Read the model definition and answer for the solid it produces. Units are mm, in the model's axes. A direction names the side the tool comes from. Give positions to 0.01 mm unless a question says otherwise; leave off trailing zeros. Order: outer loops, then holes, each group sorted by start corner. A loop starts at its lowest first (then second) coordinate and runs counter-clockwise, first axis right, second up. Notation, with made-up numbers: (-0.5, -22.75) - (15.5, -22.75) arc R16 cw to (15.5, -12.75) - close; hole circle Ø7 at (52, 12). An arc over 180 degrees is marked (long way). Use a Markdown table: item, result. Add a question column.
1. A cutting plane is placed at A-A on x = 0. Determine the outline of the cut face in (y, z) (1 decimal), and give its area (3 significant figures).
2. A cutting plane is placed at D-D on z = 0.75. Determine the outline of the cut face in (x, y) (3 decimals), and give its area (3 significant figures).
3. Which of the six approach directions +Z, -Z, +X, -X, +Y, -Y give full straight-line access (tool end or side, diameter ignored) to faces 4 (the cylindrical face through (-2.94, 0.13, -8.49)), 5 (the flat face through (-3.175, 0, -2)), 6 (the flat face through (0, 7, -3.048)), 7 (the flat face through (5, 0, 0))?
4. Consider L1, parallel to Y at x = 0, z = -1.95 (3 decimals); L2, parallel to X at y = 2, z = -2.75 (3 decimals); L3, parallel to Z at x = -3.75, y = 8.25. Determine where each line is inside the solid, lowest interval first.
5. Flat-ended cylindrical pins translate along their axes: P1, Ø3, axis at y = -1.5, z = -7.5, coming from the +X side; P2, Ø3.5, axis at x = 0, y = 6.477, coming from the +Z side; P3, Ø1, axis at x = 4.5, y = 5, coming from the -Z side. Find the tip coordinate at first contact, or state that the pin passes through.
6. For a pull along Y with two mould halves and no side action, classify faces 1 (the flat face through (0, -9.525, -4)), 2 (the cylindrical face through (2.96, 0.13, -8.48)), 3 (the cylindrical face through (-0.26, 8.46, -0.7)) as released by +Y, released by -Y, zero draft, split by the parting line, or undercut.
7. A cutting plane is placed at C-C on x = 4. Determine the outline of the cut face in (y, z) (1 decimal), and give its area (3 significant figures).
```python
from build123d import *

# Parameters (mm, degrees)
SKETCH1_W           = 12.7
SKETCH1_H           = 19.05
BOSS_EXTRUDE1_DEPTH = 1.5875
BOSS_EXTRUDE2_DEPTH = 19.05
SKETCH4_R           = 2
CUT_EXTRUDE1_DEPTH  = 4.6355


with BuildPart() as part:
    # Sketch1 → Boss-Extrude1 (new body)
    with BuildSketch(Plane.XY):
        Rectangle(SKETCH1_W, SKETCH1_H)
    extrude(amount=BOSS_EXTRUDE1_DEPTH)

    # Sketch2 → Boss-Extrude2 (add)
    with BuildSketch(Plane(origin=(0, 9.525, 0), x_dir=(1, 0, 0), z_dir=(0, 1, 0))):
        with BuildLine():
            Line((3.175, 0), (3.175, 3.048))
            Line((3.175, 3.048), (4.281466055, 3.048))
            ThreePointArc((4.281466055, 3.048), (5.652123405, 3.905760984), (5.479872098, 5.513487629))
            Line((5.479872098, 5.513487629), (3.484406043, 8.053487629))
            ThreePointArc((3.484406043, 8.053487629), (2.952239016, 8.482657351), (2.286, 8.636))
            Line((2.286, 8.636), (-2.286, 8.636))
            ThreePointArc((-2.286, 8.636), (-2.952239016, 8.482657351), (-3.484406043, 8.053487629))
            Line((-3.484406043, 8.053487629), (-5.479872098, 5.513487629))
            ThreePointArc((-5.479872098, 5.513487629), (-5.652123405, 3.905760984), (-4.281466055, 3.048))
            Line((-4.281466055, 3.048), (-3.175, 3.048))
            Line((-3.175, 3.048), (-3.175, 0))
            Line((-3.175, 0), (3.175, 0))
        make_face()
    extrude(amount=-BOSS_EXTRUDE2_DEPTH)

    # Sketch4 → Cut-Extrude1 (cut)
    with BuildSketch(Plane.XY.offset(1.5875)):
        with Locations((0, 6.477)):
            Circle(SKETCH4_R)
        with Locations((0, -6.477)):
            Circle(SKETCH4_R)
    extrude(amount=-CUT_EXTRUDE1_DEPTH, mode=Mode.SUBTRACT)


solid = part.part
```
Output values:
| question | item | result |
|---|---|---|
| 1 | outline | (-9.5, -8.6) - (9.5, -8.6) - (9.5, 1.6) - (8.5, 1.6) - (8.5, -3) - (4.5, -3) - (4.5, 1.6) - (-4.5, 1.6) - (-4.5, -3) - (-8.5, -3) - (-8.5, 1.6) - (-9.5, 1.6) - close |
| 1 | area | 158 mm² |
| 2 | outline | (-6.35, -9.525) - (6.35, -9.525) - (6.35, 9.525) - (-6.35, 9.525) - close; hole circle Ø4 at (0, -6.477); hole circle Ø4 at (0, 6.477) |
| 2 | area | 217 mm² |
| 3 | face 4 | -Z, -X, +Y, -Y |
| 3 | face 5 | -X, +Y, -Y |
| 3 | face 6 | +Z |
| 3 | face 7 | +X, +Y, -Y |
| 4 | L1 | -9.525 to -8.477, -4.477 to 4.477, 8.477 to 9.525 |
| 4 | L2 | -3.175 to 3.175 |
| 4 | L3 | -7.72 to -3.05, 0 to 1.59 |
| 5 | P1 | x = 5.1 |
| 5 | P2 | z = -3.05 |
| 5 | P3 | z = -7.4 |
| 6 | face 1 | released by -Y |
| 6 | face 2 | zero draft |
| 6 | face 3 | undercut |
| 7 | outline | (-9.5, -7.4) - (9.5, -7.4) - (9.5, -3) - (-9.5, -3) - close; (-9.5, 0) - (9.5, 0) - (9.5, 1.6) - (-9.5, 1.6) - close |
| 7 | area | 113 mm² |
